For this review, take the finished solid that the model builds, in its own axes (mm). Round coordinates to 2 decimals unless told otherwise and drop trailing zeros. Loops run counter-clockwise (first coordinate to the right, second up) from the corner with the lowest first, then second, coordinate; pieces in that order, holes last.
1. Clearance check with a flat-ended pin moving along its axis: pin 1 Ø12 at (x, z) = (-31.5, -8) entering from +Y. State where the tip first meets the part, or that it passes through.
2. Consider section A-A on y = 499.5. State the section outline as (x, z) points (3 decimals), then the cut area to 3 significant figures.
3. To check wall thickness, follow line 1 along X through (y, z) = (450, -5.5) (3 decimals); line 2 along Z through (x, y) = (-11, 505) (3 decimals); line 3 along Y through (x, z) = (-25.4, -24.7). State the ranges of each line that lie inside material, in increasing order.
4. Consider section C-C on x = -25.4. State how many separate pieces and enclosed holes the cut face has, then the cut area to 3 significant figures.
Autodesk Inventor part; units mm, degrees
ref_plane "YZ Plane" through (0, 0, 0) normal (1, 0, 0) x (0, 1, 0)
ref_plane "XZ Plane" through (0, 0, 0) normal (0, 1, 0) x (-1, 0, 0)
ref_plane "XY Plane" through (0, 0, 0) normal (0, 0, 1) x (1, 0, 0)
sketch "Sketch1" plane through (0, 0, 0) normal (0, 1, 0) x (-1, 0, 0)
  line L0 (0, 0) -> (50.8, 0)
  line L1 (50.8, 0) -> (50.8, -25.4)
  line L2 (50.8, -25.4) -> (0, -25.4)
  line L3 (0, -25.4) -> (0, 0)
  line L4 (47.625, -22.225) -> (47.625, -3.175)
  line L5 (47.625, -3.175) -> (3.175, -3.175)
  line L6 (3.175, -3.175) -> (3.175, -22.225)
  line L7 (3.175, -22.225) -> (47.625, -22.225)
  dimension "d0" = 50.8
  dimension "d1" = 25.4
  dimension "d2" = 3.175
extrude "Extrusion1" add sketch "Sketch1" along normal blind 886.206
sketch "Sketch2" plane through (-50.8, 0, 0) normal (0, 0, 1) x (1, 0, 0)
  line L0 (50.8, 0) -> (0, 0)
  line L1 (50.8, 0) -> (50.8, 886.206)
  line L2 (0, 886.206) -> (50.8, 886.206)
  line L3 (0, 0) -> (0, 886.206)
  line L4 (0, 0) -> (50.8, 0)
  line L5 (50.8, 0) -> (0, 56.4191)
  line L6 (0, 56.4191) -> (50.8, 56.4191)
  line L7 (50.8, 56.4191) -> (50.8, 0)
  line L8 (50.8, 0) -> (0, 0)
  line L9 (0, 0) -> (0, 56.4191)
  line L10 (0, 56.4191) -> (50.8, 0)
  line L11 (0, 56.4191) -> (21.859, 0)
  line L12 (47.625, 0) -> (3.175, 0)
  dimension "d5" = 48
extrude "Extrusion2" cut sketch "Sketch2" against normal blind 914.4 contours L0 L11 L5 | L11 L0 L3
sketch "Sketch3" plane through (-50.8, 886.206, 0) normal (0, 0, 1) x (1, 0, 0)
  line L0 (0, -829.7869) -> (50.8, -886.206)
  line L1 (50.8, -886.206) -> (50.8, 0)
  line L2 (0, 0) -> (50.8, 0)
  line L3 (0, -829.7869) -> (0, 0)
  line L4 (0, -829.7869) -> (50.8, -886.206)
  line L5 (0, -829.7869) -> (50.8, -778.9869)
  line L6 (50.8, -886.206) -> (50.8, 0)
  line L7 (0, -829.7869) -> (0, 0)
  line L8 (50.8, -886.206) -> (0, -886.206)
  line L9 (0, -886.206) -> (0, -923.3654)
  line L10 (0, -923.3654) -> (50.8, -923.3654)
  line L11 (50.8, -923.3654) -> (50.8, -886.206)
  dimension "d8" = 93
extrude "Extrusion3" cut sketch "Sketch3" against normal blind 25.4 contours L5 L1 L0
sketch "Sketch4" plane through (-50.8, 886.206, 0) normal (0, 0, 1) x (1, 0, 0)
  line L0 (0, -829.7869) -> (50.8, -778.9869)
  line L1 (50.8, -778.9869) -> (50.8, 0)
  line L2 (0, 0) -> (50.8, 0)
  line L3 (0, -829.7869) -> (0, 0)
  line L4 (0, 0) -> (50.8, 0)
  line L5 (0, 0) -> (50.8, 0)
  line L6 (50.8, 0) -> (50.8, -221.7928)
  line L7 (50.8, -221.7928) -> (0, -221.7928)
  line L8 (0, -221.7928) -> (0, 0)
  line L9 (0, -829.7869) -> (0, 0)
  line L10 (0, 0) -> (50.8, -50.8)
  line L11 (50.8, 0) -> (0, 0)
  line L12 (0, 0) -> (0, -56.4191)
  line L13 (0, -56.4191) -> (50.8, -56.4191)
  line L14 (50.8, -56.4191) -> (50.8, 0)
  point P0 (50.8, -886.206)
  dimension "d11" = 221.7928
  dimension "d12" = 45
  dimension "d13" = 56.4191
extrude "Extrusion4" cut sketch "Sketch4" against normal blind 25.4 contours L2 L1 L10
sketch "Sketch8" plane through (-50.8, 56.4191, 0) normal (0, 0, 1) x (1, 0, 0)
  line L0 (50.8, 778.9869) -> (0, 829.7869)
  line L1 (0, 0) -> (0, 829.7869)
  line L2 (0, 0) -> (50.8, 50.8)
  line L3 (50.8, 50.8) -> (50.8, 778.9869)
  line L4 (0, 797.6016) -> (50.8, 746.8016)
  point P0 (50.8, -56.4191)
  dimension "d24" = 22.7584
extrude "Extrusion8" cut sketch "Sketch8" against normal blind 25.4 contours L3 L4 L1 L0
sketch "Sketch9" plane through (-50.8, 56.4191, 0) normal (0, 0, 1) x (1, 0, 0)
  line L0 (50.8, 746.8016) -> (0, 797.6016)
  line L1 (0, 0) -> (0, 797.6016)
  line L2 (0, 0) -> (50.8, 50.8)
  line L3 (50.8, 50.8) -> (50.8, 746.8016)
  line L4 (0, 0) -> (0, 797.6016)
  line L5 (0, 58.228) -> (50.8, 109.028)
  line L6 (50.8, 50.8) -> (50.8, 746.8016)
  line L7 (0, 0) -> (50.8, 50.8)
  point P0 (50.8, -56.4191)
  dimension "d27" = 41.1734
extrude "Extrusion9" cut sketch "Sketch9" against normal blind 25.4 contours L3 L2 L1 L5
sketch "Sketch10" plane through (-50.8, 114.6471, 0) normal (0, 0, 1) x (1, 0, 0)
  line L0 (0, 0) -> (50.8, 50.8)
  line L1 (50.8, 50.8) -> (50.8, 688.5737)
  line L2 (50.8, 688.5737) -> (0, 739.3737)
  line L3 (0, 0) -> (0, 739.3737)
  point P0 (50.8, -114.6471)
  point P1 (25.4, 76.2)
hole "Hole1" at (-25.4, 190.8471, 0) direction (0, 0, -1) diameter 28.575 end through all
sketch "Sketch11" plane through (-50.8, 114.6471, 0) normal (0, 0, 1) x (1, 0, 0)
  circle A0 centre (25.4, 76.2) radius 14.2875
  line L0 (0, 0) -> (50.8, 50.8)
  line L1 (50.8, 50.8) -> (50.8, 688.5737)
  line L2 (50.8, 688.5737) -> (0, 739.3737)
  line L3 (0, 0) -> (0, 739.3737)
  point P0 (50.8, -114.6471)
  point P1 (25.4, 431.8)
  dimension "d37" = 355.6
hole "Hole2" at (-25.4, 546.4471, 0) direction (0, 0, -1) diameter 28.575 end through all
sketch "Sketch12" plane through (-50.8, 114.6471, 0) normal (0, 0, 1) x (1, 0, 0)
  circle A0 centre (25.4, 431.8) radius 14.2875
  circle A1 centre (25.4, 76.2) radius 14.2875
  line L0 (50.8, 50.8) -> (0, 0)
  line L1 (0, 0) -> (0, 739.3737)
  line L2 (0, 739.3737) -> (50.8, 688.5737)
  line L3 (50.8, 50.8) -> (50.8, 688.5737)
  line L4 (50.8, 50.8) -> (50.8, 688.5737)
  line L5 (50.8, 688.5737) -> (29.7688, 688.5737)
  line L6 (29.7688, 688.5737) -> (29.7688, 709.6049)
  line L7 (29.7688, 709.6049) -> (50.8, 709.6049)
  line L8 (50.8, 709.6049) -> (50.8, 688.5737)
  line L9 (50.8, 709.6049) -> (0, 658.8049)
  line L10 (0, 0) -> (0, 739.3737)
  line L11 (0, 658.8049) -> (50.8, 658.8049)
  line L12 (50.8, 658.8049) -> (50.8, 739.3737)
  line L13 (50.8, 739.3737) -> (0, 739.3737)
  line L14 (0, 739.3737) -> (0, 658.8049)
  line L15 (0, 739.3737) -> (50.8, 688.5737)
  line L16 (50.8, 709.6049) -> (29.7688, 688.5737)
  line L17 (50.8, 688.5737) -> (50.8, 709.6049)
  line L18 (29.7688, 688.5737) -> (50.8, 688.5737)
  point P0 (50.8, -114.6471)
  dimension "d45" = 21.0312
  dimension "d46" = 21.0312
  dimension "d47" = 50.8
  dimension "d48" = 80.5688
  dimension "d49" = 50.8
extrude "Extrusion10" add sketch "Sketch12" against normal blind 25.4 contours L5 L9 L2 | L2 L9 L8
extrude "Extrusion11" cut sketch "Sketch12" against normal blind 25.4 contours L1 L2 L6 L9 | L13 L12 L7 L2
sketch "Sketch14" plane through (0, 165.4471, -25.4) normal (0, 0, -1) x (-1, 0, 0)
  circle A0 centre (25.4, 381) radius 14.2875
  circle A1 centre (25.4, 25.4) radius 14.2875
  line L0 (50.8, 608.0049) -> (21.0312, 637.7737)
  line L1 (21.0312, 637.7737) -> (21.0312, 658.8049)
  line L2 (21.0312, 658.8049) -> (10.5156, 648.2893)
  line L3 (10.5156, 648.2893) -> (0, 658.8049)
  line L4 (0, 0) -> (0, 658.8049)
  line L5 (0, 0) -> (50.8, -50.8)
  line L6 (50.8, -50.8) -> (50.8, 608.0049)
  line L7 (10.5156, 648.2893) -> (21.0312, 637.7737)
  line L8 (21.0312, 637.7737) -> (47.625, 611.1799)
  line L9 (21.0312, 637.7737) -> (21.0312, 658.8049)
  line L10 (21.0312, 658.8049) -> (21.0312, 637.7737)
  line L11 (10.5156, 648.2893) -> (21.0312, 658.8049)
  point P0 (0, -165.4471)
extrude "Extrusion12" cut sketch "Sketch14" against normal through all contours L7 L2 L1
sketch "Sketch15" plane through (0, 0, 0) normal (0, 1, 0) x (-1, 0, 0)
  line L0 (47.625, -22.225) -> (3.175, -22.225)
  line L1 (3.175, -3.175) -> (47.625, -3.175)
  line L2 (47.625, -3.175) -> (47.625, -22.225)
  line L3 (3.175, -22.225) -> (3.175, -3.175)
  point P0 (0, 0)
extrude "Extrusion13" cut sketch "Sketch15" along normal blind 2540
sketch "Sketch16" plane through (0, 165.4471, -25.4) normal (0, 0, -1) x (-1, 0, 0)
  line L0 (50.8, 608.0049) -> (0, 658.8049)
  line L1 (0, 0) -> (0, 658.8049)
  line L2 (0, 0) -> (50.8, -50.8)
  line L3 (50.8, -50.8) -> (50.8, 608.0049)
  circle A0 centre (25.4, 25.4) radius 14.2875
  circle A1 centre (25.4, 381) radius 14.2875
  line L4 (50.8, 608.0049) -> (-0.2406, 608.0049)
  line L5 (11.1125, 647.6924) -> (15.4769, 652.0568)
  line L6 (50.8, 616.7337) -> (-0.2406, 667.7743)
  line L7 (47.625, 611.1799) -> (3.175, 655.6299)
  line L8 (0, 658.8049) -> (0, 667.5337)
  line L9 (0, 658.8049) -> (50.8, 608.0049)
  line L10 (50.8, 608.0049) -> (50.8, 616.7337)
  line L11 (0, 658.8049) -> (50.8, 608.0049)
  point P0 (0, -165.4471)
  dimension "d58" = 6.1722
  dimension "d59" = 90
  dimension "d60" = 8.7288
extrude "Extrusion14" add sketch "Sketch16" against normal blind 25.4 contours L0 L5 L6 L10 | L0 L8 L6 L5
sketch "Sketch17" plane through (0, 0, 0) normal (0, 1, 0) x (-1, 0, 0)
  line L0 (47.625, -3.175) -> (3.175, -3.175)
  line L1 (47.625, -22.225) -> (47.625, -3.175)
  line L2 (47.625, -22.225) -> (3.175, -22.225)
  line L3 (3.175, -22.225) -> (3.175, -3.175)
  point P0 (0, 0)
extrude "Extrusion15" cut sketch "Sketch17" along normal blind 2540
sketch "Sketch18" plane through (-50.8, 114.6471, 0) normal (0, 0, 1) x (1, 0, 0)
  circle A0 centre (25.4, 431.8) radius 14.2875
  circle A1 centre (25.4, 431.8) radius 14.2875
  circle A2 centre (25.4, 641.35) radius 14.2875
  point P0 (50.8, -114.6471)
  dimension "d65" = 28.575
  dimension "d66" = 209.55
extrude "Extrusion16" cut sketch "Sketch18" against normal blind 25.4 contours A2
properties part number "AngleBrace.ver2-1111-2020" material "Aluminum 6061"
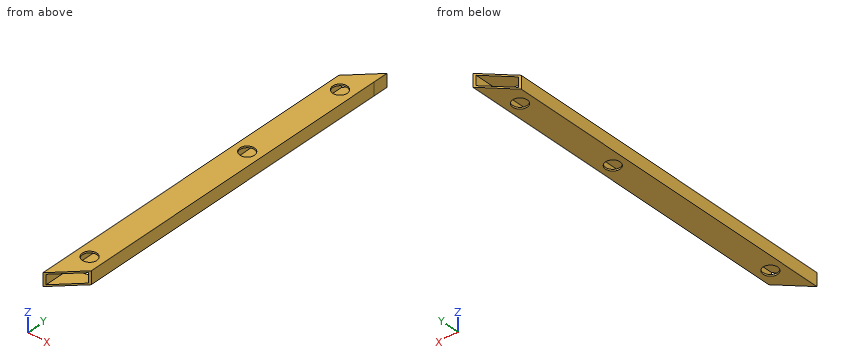
Resolved:
1. pin 1: stops at y = 805.05
2. outline: (-50.8, -25.4) - (0, -25.4) - (0, 0) - (-50.8, 0) - close; hole (-47.625, -22.225) - (-3.175, -22.225) - (-3.175, -3.175) - (-47.625, -3.175) - close
2. area: 444 mm2
3. line 1: x = -50.8 to -47.625, -3.175 to 0
3. line 2: z = -25.4 to -22.225, -3.175 to 0
3. line 3: y = 140.05 to 176.56, 205.13 to 532.16, 560.73 to 741.71, 770.28 to 807.58
4. separate pieces: 8
4. enclosed holes: 0
4. area: 3,690 mm2
